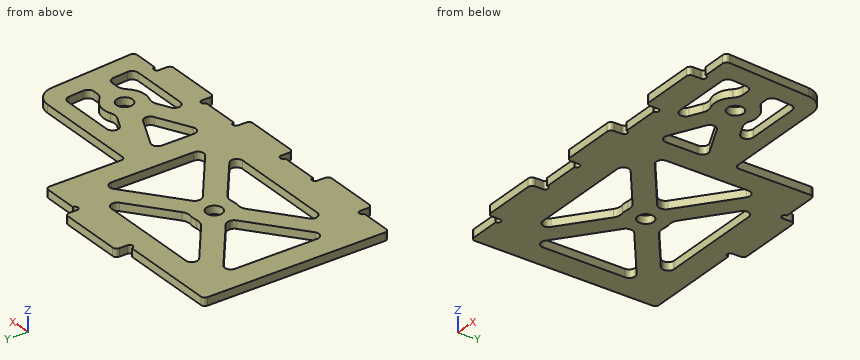
from build123d import *

# Parameters (mm, degrees)
EXTRUDE_1_DEPTH     = 2
SKETCH_2_R          = 0.75
SKETCH_2_W          = 43
SKETCH_2_H          = 33
CUT_EXTRUDE_1_DEPTH = 102.422384117
EXTRUDE_START       = -2
EXTRUDE_1_2_DEPTH   = 2
FILLET_1_R          = 1
SKETCH_4_R          = 2
CUT_EXTRUDE_2_DEPTH = 102.422384117
FILLET_2_R          = 3
FILLET_3_R          = 1.5


# Read off the part's stored shape, not the designer's step: 拉伸-薄壁1
with BuildPart() as part:
    # 草图1 → Extrude 1 (new body)
    with BuildSketch(Plane.XY):
        with BuildLine():
            Line((88.497370929, 1.072465371), (86.986854645, 21.862326856))
            ThreePointArc((86.986854645, 21.862326856), (85.405023181, 25.161395518), (82, 26.5))
            Line((82, 26.5), (55, 26.5))
            Line((55, 26.5), (55, 46.5))
            Line((55, 46.5), (44, 46.5))
            Line((44, 46.5), (44, 49.5))
            Line((44, 49.5), (26.5, 49.5))
            Line((26.5, 49.5), (26.5, 46.5))
            Line((26.5, 46.5), (0, 46.5))
            Line((0, 46.5), (0, 0))
            Line((0, 0), (10, 0))
            Line((10, 0), (10, -3))
            Line((10, -3), (25, -3))
            Line((25, -3), (25, 0))
            Line((25, 0), (37.5, 0))
            Line((37.5, 0), (37.5, -3))
            Line((37.5, -3), (52.5, -3))
            Line((52.5, -3), (52.5, 0))
            Line((52.5, 0), (65, 0))
            Line((65, 0), (65, -3))
            Line((65, -3), (80, -3))
            Line((80, -3), (80, 0))
            Line((80, 0), (87.5, 0))
            ThreePointArc((87.5, 0), (88.232279104, 0.318995364), (88.497370929, 1.072465371))
        make_face()
    extrude(amount=EXTRUDE_1_DEPTH)

    # 草图2 → 切除-拉伸1 (cut, through all)
    with BuildSketch(Plane.XY.offset(2)):
        with Locations((9.25, 0)):
            Circle(SKETCH_2_R)
        with Locations((25.75, 0)):
            Circle(SKETCH_2_R)
        with Locations((36.75, 0)):
            Circle(SKETCH_2_R)
        with Locations((53.25, 0)):
            Circle(SKETCH_2_R)
        with Locations((64.25, 0)):
            Circle(SKETCH_2_R)
        with Locations((80.75, 0)):
            Circle(SKETCH_2_R)
        with Locations((25.75, 46.5)):
            Circle(SKETCH_2_R)
        with Locations((44.75, 46.5)):
            Circle(SKETCH_2_R)
        with Locations((27.5, 24)):
            Rectangle(SKETCH_2_W, SKETCH_2_H)
        Polygon((55, 4), (83.271486825, 4), (81.92734361, 22.5), (55, 22.5), align=None)
    extrude(amount=-CUT_EXTRUDE_1_DEPTH, mode=Mode.SUBTRACT)

    # Extrude 1 2 outline → Extrude 1 2 (add)
    with BuildSketch(Plane.XY.offset(2).offset(EXTRUDE_START)):
        with BuildLine():
            Line((55, 19.707975069), (67.987198163, 13.25))
            Line((67.987198163, 13.25), (55, 6.792024931))
            Line((55, 6.792024931), (55, 4))
            Line((55, 4), (60.614853056, 4))
            Line((60.614853056, 4), (70.581480185, 8.955975008))
            ThreePointArc((70.581480185, 8.955975008), (74.80264095, 8.139120986), (78.218597547, 10.75))
            Line((78.218597547, 10.75), (82.781056192, 10.75))
            Line((82.781056192, 10.75), (82.417774242, 15.75))
            Line((82.417774242, 15.75), (78.218597547, 15.75))
            ThreePointArc((78.218597547, 15.75), (74.80264095, 18.360879014), (70.581480185, 17.544024992))
            Line((70.581480185, 17.544024992), (60.614853056, 22.5))
            Line((60.614853056, 22.5), (55, 22.5))
            Line((55, 22.5), (55, 19.707975069))
        make_face()
        with BuildLine():
            Line((22.315603781, 23.172633188), (6, 10.651355868))
            Line((6, 10.651355868), (6, 7.5))
            Line((6, 7.5), (10.106312192, 7.5))
            Line((10.106312192, 7.5), (25.359697706, 19.206086558))
            ThreePointArc((25.359697706, 19.206086558), (27.5, 18.75), (29.640302294, 19.206086558))
            Line((29.640302294, 19.206086558), (44.893687808, 7.5))
            Line((44.893687808, 7.5), (49, 7.5))
            Line((49, 7.5), (49, 10.651355868))
            Line((49, 10.651355868), (32.684396219, 23.172633188))
            ThreePointArc((32.684396219, 23.172633188), (32.75, 24), (32.684396219, 24.827366812))
            Line((32.684396219, 24.827366812), (49, 37.348644132))
            Line((49, 37.348644132), (49, 40.5))
            Line((49, 40.5), (44.893687808, 40.5))
            Line((44.893687808, 40.5), (29.640302294, 28.793913442))
            ThreePointArc((29.640302294, 28.793913442), (27.5, 29.25), (25.359697706, 28.793913442))
            Line((25.359697706, 28.793913442), (10.106312192, 40.5))
            Line((10.106312192, 40.5), (6, 40.5))
            Line((6, 40.5), (6, 37.348644132))
            Line((6, 37.348644132), (22.315603781, 24.827366812))
            ThreePointArc((22.315603781, 24.827366812), (22.25, 24), (22.315603781, 23.172633188))
        make_face()
    extrude(amount=EXTRUDE_1_2_DEPTH)

    # 圆角1
    fillet_1_edges = [part.edges().sort_by_distance(p)[0] for p in [
        (52.5, -3, 1),
        (37.5, -3, 1),
        (25, -3, 1),
        (10, -3, 1),
        (0, 0, 1),
        (0, 46.5, 1),
        (26.5, 49.5, 1),
        (44, 49.5, 1),
        (55, 46.5, 1),
        (55, 26.5, 1),
        (80, -3, 1),
        (65, -3, 1),
    ]]
    fillet(fillet_1_edges, radius=FILLET_1_R)

    # 草图4 → 切除-拉伸2 (cut, through all)
    with BuildSketch(Plane.XY.offset(2)):
        with Locations((27.5, 24)):
            Circle(SKETCH_4_R)
        with Locations((73.602051219, 13.25)):
            Circle(SKETCH_4_R)
    extrude(amount=-CUT_EXTRUDE_2_DEPTH, mode=Mode.SUBTRACT)

    # 圆角2
    fillet_2_edges = [part.edges().sort_by_distance(p)[0] for p in [
        (70.581480185, 17.544024992, 1),
        (78.218597547, 15.75, 1),
        (70.581480185, 8.955975008, 1),
        (78.218597547, 10.75, 1),
        (29.640302294, 28.793913442, 1),
        (25.359697706, 28.793913442, 1),
        (29.640302294, 19.206086558, 1),
        (25.359697706, 19.206086558, 1),
    ]]
    fillet(fillet_2_edges, radius=FILLET_2_R)

    # 圆角3
    fillet_3_edges = [part.edges().sort_by_distance(p)[0] for p in [
        (81.92734361, 22.5, 1),
        (83.271486825, 4, 1),
        (60.614853056, 4, 1),
        (82.417774242, 15.75, 1),
        (82.781056192, 10.75, 1),
        (60.614853056, 22.5, 1),
        (55, 19.707975069, 1),
        (55, 6.792024931, 1),
        (67.987198163, 13.25, 1),
        (10.106312192, 7.5, 1),
        (44.893687808, 7.5, 1),
        (49, 37.348644132, 1),
        (49, 10.651355868, 1),
        (10.106312192, 40.5, 1),
        (44.893687808, 40.5, 1),
        (6, 37.348644132, 1),
        (6, 10.651355868, 1),
        (22.315603781, 23.172633188, 1),
        (32.684396219, 23.172633188, 1),
        (32.684396219, 24.827366812, 1),
        (22.315603781, 24.827366812, 1),
    ]]
    fillet(fillet_3_edges, radius=FILLET_3_R)


solid = part.part
Check sheet for the modelled part. Datum: model origin and axes. Units: mm. Give positions to 0.01 mm unless a question says otherwise; leave off trailing zeros. Loops run counter-clockwise (first coordinate to the right, second up) from the corner with the lowest first, then second, coordinate; pieces in that order, holes last. Notation, with made-up numbers: M -2,79.25 L 54,79.25 A29 cw 54,115.25 Z; hole C 42,38.5 d1. An arc over 180 degrees is marked long. Return JSON: item names as keys, results as strings. Group by question number.
1. Go/stop test with flat-tipped pins: pin 1 (1 mm diameter, centred on y = 26, z = 1.5, fed in from +X); pin 2 (0.5 mm diameter, centred on x = 81, z = 0.5, fed in from -Y); pin 3 (1.2 mm diameter, centred on x = 80.5, z = 1.5, fed in from +Y). Record where each tip stops, or that it passes through.
2. Cross-section at A-A on x = 39.5. Record the boundary of the cut face in (y, z).
3. Cross-section at B-B on z = 0.55. State how many separate pieces and enclosed holes the cut face has, plus the area to 3 significant figures.
4. Thickness scan on L1, parallel to Y at x = 58, z = 1.35; L2, parallel to Y at x = 34.5, z = 1.4; L3, parallel to X at y = 21, z = 0.4. Record the ranges inside material, lowest first.
Return value:
{
 "1": {"pin 1": "x = 85", "pin 2": "y = 0.56", "pin 3": "y = 26.5"},
 "2": {"outline": "M -3,0 L 7.5,0 L 7.5,2 L -3,2 Z; M 11.64,0 L 17.94,0 L 17.94,2 L 11.64,2 Z; M 30.06,0 L 36.36,0 L 36.36,2 L 30.06,2 Z; M 40.5,0 L 49.5,0 L 49.5,2 L 40.5,2 Z"},
 "3": {"separate pieces": "1", "enclosed holes": "9", "area": "2,440 mm^2"},
 "4": {"L1": "0 to 8.28, 18.22 to 26.5", "L2": "0 to 7.5, 15.48 to 21.78, 26.22 to 32.52, 40.5 to 49.5", "L3": "0 to 6, 19.48 to 35.52, 49 to 65.5, 82.04 to 87.05"}
}
